from build123d import *

# Parameters (mm, degrees)
SKETCH2_W               = 10
SKETCH2_H               = 1
FILLET3_RADIUS          = 5
FILLET3_LENGTH          = 1
FILLET4_RADIUS          = 5
FILLET4_LENGTH          = 1
CUT_EXTRUDE1_DEPTH      = 41.51542916
CUT_EXTRUDE1_DEPTH_BACK = 41.51542916
SKETCH3_R               = 1.5


with BuildPart() as part:
    # Sweep1: sweep along a path in Sketch1
    with BuildLine(Plane(origin=(0, 0, 0), x_dir=(0, 0, -1), z_dir=(1, 0, 0))) as sweep1_path:
        Line((0, 0), (11.25, 0))
        Line((11.25, 0), (11.25, -6))
        ThreePointArc((11.25, -6), (18.75, -13.5), (26.25, -6))
        Line((26.25, -6), (26.25, 0))
        Line((26.25, 0), (37.5, 0))
    # Sketch2 → Sweep1 (sweep)
    with BuildSketch(Plane.XY):
        with Locations((0, -0.5)):
            Rectangle(SKETCH2_W, SKETCH2_H)
    sweep(path=sweep1_path.line, transition=Transition.RIGHT)

    # Fillet3: full round fillet: the end face becomes a half cylinder, R = half its width
    fillet3_face = Plane((0, -0.5, 0), x_dir=(0, -1, 0), z_dir=(0, 0, 1))  # on the end face: x along it, z out of the body
    fillet3_slab = fillet3_face.offset(-FILLET3_RADIUS / 2) * Box(FILLET3_LENGTH, 2 * FILLET3_RADIUS, FILLET3_RADIUS, mode=Mode.PRIVATE)  # the body's end, R deep
    fillet3_round = Plane((0, -0.5, -5), x_dir=(0, 0, 1), z_dir=(0, -1, 0)) * Cylinder(FILLET3_RADIUS, FILLET3_LENGTH, mode=Mode.PRIVATE)  # its axis R under the face
    add(fillet3_slab - fillet3_round, mode=Mode.SUBTRACT)

    # Fillet4: full round fillet: the end face becomes a half cylinder, R = half its width
    fillet4_face = Plane((0, -0.5, -37.5), x_dir=(0, 1, 0), z_dir=(0, 0, -1))  # on the end face: x along it, z out of the body
    fillet4_slab = fillet4_face.offset(-FILLET4_RADIUS / 2) * Box(FILLET4_LENGTH, 2 * FILLET4_RADIUS, FILLET4_RADIUS, mode=Mode.PRIVATE)  # the body's end, R deep
    fillet4_round = Plane((0, -0.5, -32.5), x_dir=(0, 0, -1), z_dir=(0, 1, 0)) * Cylinder(FILLET4_RADIUS, FILLET4_LENGTH, mode=Mode.PRIVATE)  # its axis R under the face
    add(fillet4_slab - fillet4_round, mode=Mode.SUBTRACT)

    # Sketch3 → Cut-Extrude1 (cut, two sides: drawn at the far end of the back side and taken through both)
    with BuildSketch(Plane(origin=(0, 0, 0), x_dir=(1, 0, 0), z_dir=(0, 1, 0)).offset(-CUT_EXTRUDE1_DEPTH_BACK)):
        with Locations(Location((0, 5, 0), (0, 0, 270))):
            Circle(SKETCH3_R)
        with Locations(Location((0, 32.5, 0), (0, 0, 270))):
            Circle(SKETCH3_R)
    extrude(amount=CUT_EXTRUDE1_DEPTH + CUT_EXTRUDE1_DEPTH_BACK, mode=Mode.SUBTRACT)


solid = part.part
Work out the finished part from the listing and answer in its coordinate system (mm). A direction names the side the tool comes from. Give positions to 0.01 mm unless a question says otherwise; leave off trailing zeros. Loops run counter-clockwise (first coordinate to the right, second up) from the corner with the lowest first, then second, coordinate; pieces in that order, holes last. Notation, with made-up numbers: (31, -10.75) - (65, -10.75) arc R29 cw to (65, 21.25) - close; hole circle Ø4 at (-30.5, 89.5). An arc over 180 degrees is marked (long way). Answer in a Markdown table with one row per item. Add a question column.
Q1. The part is cut by section A-A (x = 0). Determine the outline of the cut face in (y, z), and give its area (3 significant figures).
Q2. Consider line 1 along Z through (x, y) = (0, -0.4); line 2 along X through (y, z) = (-0.55, -32.5); line 3 along Z through (x, y) = (4, -4.5). Determine where each line is inside the solid, lowest interval first.
Q3. Each of these flat-tipped pins is pushed along its axis until it touches: P1, Ø5, axis at x = -0.5, z = -5, coming from the -Y side; P2, Ø1.5, axis at x = 1, y = -4, coming from the +Z side; P3, Ø5, axis at x = 1, z = -19, coming from the +Y side. Where does it stop, or does it pass through?
Q4. The part is cut by section D-D (z = -33.5). Determine the outline of the cut face in (x, y), and give its area (3 significant figures).
Q5. The part is cut by section C-C (x = 4). Determine the outline of the cut face in (y, z), and give its area (3 significant figures).
Q6. A tool of negligible diameter and unlimited length cuts with its end or side. For faces 5 (the flat face through (0, -3, -26.25)), 6 (the flat face through (1, -1, -31)), 7 (the flat face through (0, -4, -10.25)), 8 (the flat face through (-5, -14, -19)), from which of +Z, -Z, +X, -X, +Y, -Y can it reach the whole face along a straight path? Write none if from no direction.
Q7. The part is cut by section B-B (y = -5.25). Determine the outline of the cut face in (x, z), and give its area (3 significant figures).
Q8. Determine the mould class of faces 1 (the flat face through (0, 0, -7)), 2 (the cylindrical face through (-0.1, -13.5, -18.6)), 3 (the flat face through (0, -3, -27.25)), 4 (the flat face through (0, -3, -11.25)) for opening direction Z: released by +Z, released by -Z, zero draft, split by the parting line, or undercut.
Solution:
| question | item | result |
|---|---|---|
| 1 | outline | (-6, -27.25) - (-1, -27.25) - (-1, -31) - (0, -31) - (0, -26.25) - (-6, -26.25) arc R7.5 cw to (-6, -11.25) - (0, -11.25) - (0, -6.5) - (-1, -6.5) - (-1, -10.25) - (-6, -10.25) arc R8.5 ccw to start; (-1, -37.5) - (0, -37.5) - (0, -34) - (-1, -34) - close; (-1, -3.5) - (0, -3.5) - (0, 0) - (-1, 0) - close |
| 1 | area | 51.6 mm² |
| 2 | line 1 | z = -37.5 to -34, -31 to -26.25, -11.25 to -6.5, -3.5 to 0 |
| 2 | line 2 | x = -5 to -1.5, 1.5 to 5 |
| 2 | line 3 | z = -27.25 to -26.25, -11.25 to -10.25 |
| 3 | P1 | stops at y = -1 |
| 3 | P2 | stops at z = -10.25 |
| 3 | P3 | stops at y = -12.98 |
| 4 | outline | (-4.9, -1) - (-1.12, -1) - (-1.12, 0) - (-4.9, 0) - close; (1.12, -1) - (4.9, -1) - (4.9, 0) - (1.12, 0) - close |
| 4 | area | 7.56 mm² |
| 5 | outline | (-6, -27.25) - (-1, -27.25) - (-1, -35.5) - (0, -35.5) - (0, -26.25) - (-6, -26.25) arc R7.5 cw to (-6, -11.25) - (0, -11.25) - (0, -2) - (-1, -2) - (-1, -10.25) - (-6, -10.25) arc R8.5 ccw to start |
| 5 | area | 53.6 mm² |
| 6 | face 5 | +X, -X, +Y |
| 6 | face 6 | -Z, +X, -X, -Y |
| 6 | face 7 | +Z, +X, -X, -Y |
| 6 | face 8 | +Z, -Z, -X, +Y, -Y |
| 7 | outline | (-5, -27.25) - (5, -27.25) - (5, -26.25) - (-5, -26.25) - close; (-5, -11.25) - (5, -11.25) - (5, -10.25) - (-5, -10.25) - close |
| 7 | area | 20.0 mm² |
| 8 | face 1 | zero draft |
| 8 | face 2 | undercut |
| 8 | face 3 | released by -Z |
| 8 | face 4 | undercut |
